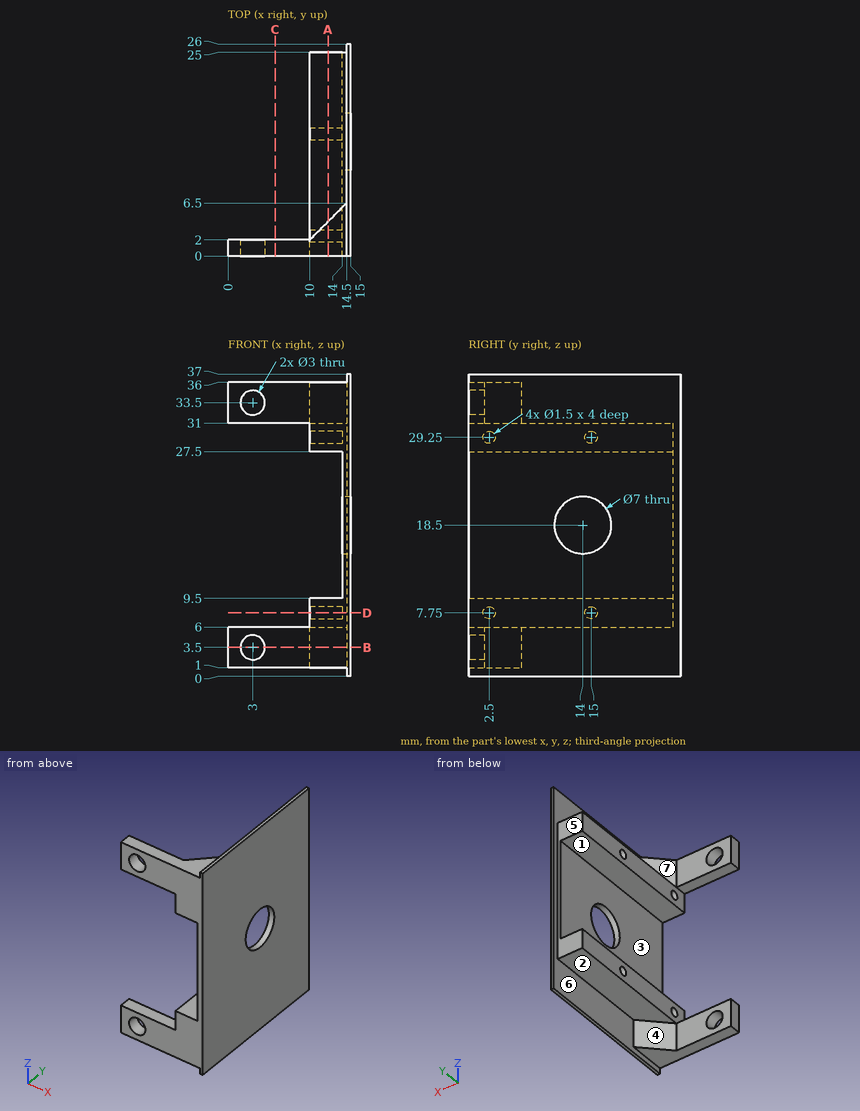
Source: three-view drawing plus pictorial views. Frame: mm from the lowest corner of the part. A direction names the side the tool comes from. Coordinates: 2 decimals unless noted, no trailing zeros. Write each loop counter-clockwise with the first axis right and the second up, starting at its lowest first coordinate (ties: lowest second). Pieces come first, ordered by that corner, then holes. Notation, with made-up numbers: (53, 42) - (68, 42) arc R16 cw to (68, 47) - close; hole circle Ø11 at (-29, 39). An arc over 180 degrees is marked (long way). Return JSON: item names as keys, results as strings.
Item 1: Reachability of the marked faces 5, 6 and 7 from +Z, -Z, +X, -X, +Y, -Y: full face, straight path, thin tool, end or side. Return the list, or none.
Completed:
{"face 5": "+Z, -Z, -X, +Y", "face 6": "-X, +Y", "face 7": "+Z, -X, +Y"}
Item 2: Section query D-D (z = 7.75). Output: boundary loops of the cut face in (x, y).
Completed:
{"outline": "(10, 0) - (15, 0) - (15, 26) - (14.5, 26) - (14.5, 25) - (10, 25) - (10, 15.75) - (14, 15.75) - (14, 14.25) - (10, 14.25) - (10, 3.25) - (14, 3.25) - (14, 1.75) - (10, 1.75) - close"}
Item 3: Pin query (flat end, axial travel): pin 1 Ø1.6 at (y, z) = (15, 8) entering from -X; pin 2 Ø6 at (x, y) = (6, 23) entering from -Z; pin 3 Ø0.6 at (x, y) = (3, 1.5) entering from +Z; pin 4 Ø2 at (x, y) = (12, 18.5) entering from -Z. Return the tip coordinate at first contact, or that it passes through.
Completed:
{"pin 1": "stops at x = 10", "pin 2": "passes through", "pin 3": "stops at z = 36", "pin 4": "stops at z = 6"}
Item 4: Section query A-A (x = 12.25). Output: boundary loops of the cut face in (y, z), and give its area (3 significant figures).
Completed:
{"outline": "(0, 1) - (4.25, 1) - (4.25, 6) - (25, 6) - (25, 9.5) - (0, 9.5) - close; (0, 27.5) - (25, 27.5) - (25, 31) - (4.25, 31) - (4.25, 36) - (0, 36) - close; hole circle Ø1.5 at (2.5, 7.75); hole circle Ø1.5 at (2.5, 29.25); hole circle Ø1.5 at (15, 7.75); hole circle Ø1.5 at (15, 29.25)", "area": "210 mm2"}
Item 5: Pull-direction query (Z, two-part tool) for the marked faces 1, 2, 3 and 4; classes: +Z half, -Z half, draft (parallel to the pull), parting line (faces both ways), or undercut.
Completed:
{"face 1": "undercut", "face 2": "-Z half", "face 3": "undercut", "face 4": "draft"}
Item 6: Section query C-C (x = 5.75). Output: boundary loops of the cut face in (y, z), and give its area (3 significant figures).
Completed:
{"outline": "(0, 1) - (2, 1) - (2, 6) - (0, 6) - close; (0, 31) - (2, 31) - (2, 36) - (0, 36) - close", "area": "20.0 mm2"}
Item 7: Line query: L1, parallel to Z at x = 3, y = 0.8; L2, parallel to Y at x = 11.75, z = 29.25; L3, parallel to Y at x = 14.3, z = 18.5. Output: solid intervals per line, ascending.
Completed:
{"L1": "z = 1 to 2, 5 to 6, 31 to 32, 35 to 36", "L2": "y = 0 to 1.75, 3.25 to 14.25, 15.75 to 25", "L3": "y = 0 to 10.5, 17.5 to 25"}
Item 8: Section query B-B (z = 3.5). Output: boundary loops of the cut face in (x, y), and give its area (3 significant figures).
Completed:
{"outline": "(0, 0) - (1.5, 0) - (1.5, 2) - (0, 2) - close; (4.5, 0) - (15, 0) - (15, 26) - (14.5, 26) - (14.5, 6.5) - (10, 2) - (4.5, 2) - close", "area": "46.1 mm2"}
